from build123d import *

# Parameters (mm, degrees)
F0_W     = 101.6
F0_H     = 184.15
F0_R     = 15.748
F0_W_2   = 12.7
F0_H_2   = 19.3294
F1_DEPTH = 16.764


with BuildPart() as f1:
    # F0 (on Front) → F1 (new body)
    with BuildSketch(Plane.XZ):
        with Locations((0, 5.400208)):
            Rectangle(F0_W, F0_H)
        with Locations((0, -10.347792)):
            Circle(F0_R, mode=Mode.SUBTRACT)
        with Locations((18.5166, -67.243792)):
            Circle(F0_R, mode=Mode.SUBTRACT)
        with Locations((-18.8849, 63.121708)):
            Rectangle(F0_W_2, F0_H_2, mode=Mode.SUBTRACT)
        with Locations((18.5166, 63.121708)):
            Rectangle(F0_W_2, F0_H_2, mode=Mode.SUBTRACT)
    extrude(amount=F1_DEPTH)


solid = f1.part
Geometry: final body of the model. Coordinates: model frame, mm. A direction names the side the tool comes from. Give positions to 0.01 mm unless a question says otherwise; leave off trailing zeros. Loops run counter-clockwise (first coordinate to the right, second up) from the corner with the lowest first, then second, coordinate; pieces in that order, holes last. Notation, with made-up numbers: (31, -22.75) - (85, -22.75) arc R7 cw to (85, -15.75) - close; hole circle Ø4 at (-39, 89.5). An arc over 180 degrees is marked (long way). One line per question, with ' | ' between items. Start each with the question number.
(1) Pull-direction query (Z, two-part tool) for faces 3 (the flat face through (-1, -8, 97.475)), 4 (the flat face through (-1, -8, -86.675)), 5 (the flat face through (18, -8, 53.457)); classes: released by +Z, released by -Z, zero draft, split by the parting line, or undercut.
(2) Section query C-C on y = -6.75. Return loops of the section in (x, z).
(3) Section query A-A on x = 0. Return loops of the section in (y, z).
(4) Section query D-D on x = 31.5. Return loops of the section in (y, z), then the cut area to 3 significant figures.
(5) Reachability of faces 1 (the flat face through (-1, 0, 7)), 2 (the flat face through (12.167, -8, 63)) from +Z, -Z, +X, -X, +Y, -Y: full face, straight path, thin tool, end or side. Return the list, or none.
(6) Section query B-B on x = 19. Return loops of the section in (y, z), then the cut area to 3 significant figures.
(7) Contact query for a flat-ended pin moving along its axis: pin 1 (25 mm diameter, centred on x = 18.52, z = -67.24, fed in from -Y). Output: stop coordinate, or through.
(8) Ray query, line 1 (X direction, y = -11, z = 69); line 2 (Z direction, x = 22.5, y = -16); line 3 (Z direction, x = -21, y = -7.5). Return the intervals inside material, ascending. Write a range as from..to.
The answers:
1) face 3: released by +Z | face 4: released by -Z | face 5: undercut
2) outline: (-50.8, -86.67) - (50.8, -86.67) - (50.8, 97.48) - (-50.8, 97.48) - close; hole (-25.23, 53.46) - (-12.53, 53.46) - (-12.53, 72.79) - (-25.23, 72.79) - close; hole circle Ø31.5 at (0, -10.35); hole circle Ø31.5 at (18.52, -67.24); hole (12.17, 53.46) - (24.87, 53.46) - (24.87, 72.79) - (12.17, 72.79) - close
3) outline: (-16.76, -86.67) - (0, -86.67) - (0, -26.1) - (-16.76, -26.1) - close; (-16.76, 5.4) - (0, 5.4) - (0, 97.48) - (-16.76, 97.48) - close
4) outline: (-16.76, -86.67) - (0, -86.67) - (0, -76.16) - (-16.76, -76.16) - close; (-16.76, -58.33) - (0, -58.33) - (0, 97.48) - (-16.76, 97.48) - close | area: 2,790 mm2
5) face 1: +Z, -Z, +X, -X, +Y | face 2: +Y, -Y
6) outline: (-16.76, -86.67) - (0, -86.67) - (0, -82.98) - (-16.76, -82.98) - close; (-16.76, -51.5) - (0, -51.5) - (0, 53.46) - (-16.76, 53.46) - close; (-16.76, 72.79) - (0, 72.79) - (0, 97.48) - (-16.76, 97.48) - close | area: 2,240 mm2
7) pin 1: through
8) line 1: -50.8..-25.23, -12.53..12.17, 24.87..50.8 | line 2: -86.67..-82.48, -52.01..53.46, 72.79..97.48 | line 3: -86.67..53.46, 72.79..97.48
